Here's how the part is built. I have some questions about the finished solid (model axes, mm). A direction names the side the tool comes from. Round coordinates to 2 decimals unless told otherwise and drop trailing zeros. Write each loop counter-clockwise with the first axis right and the second up, starting at its lowest first coordinate (ties: lowest second). Pieces come first, ordered by that corner, then holes. Notation, with made-up numbers: (55, 34.5) - (80, 34.5) arc R24 ccw to (80, 72.5) - close; hole circle Ø4 at (3.5, 41.5). An arc over 180 degrees is marked (long way). Use one line per item in the form item = value. Start each with the question number.
1. I want a section at C-C, the plane x = -31. List the corners of the cut face in (y, z) for me.
2. We'd pull the mould along X, two halves only. Please class faces 5 (the flat face through (-12.7, -157, 6)), 6 (the flat face through (-159, -52.032, 6)), 7 (the cylindrical face through (-122.91, 115.86, 6.26)): +X half, -X half, draft (parallel to the pull), parting line (faces both ways), or undercut.
3. I want a section at A-A, the plane z = 5.25. List the corners of the cut face in (x, y) for me.
4. Which directions (+Z, -Z, +X, -X, +Y, -Y) give clear straight access to the entire face, cutting with the end or side of a thin tool? Please do faces 1 (the cylindrical face through (-9.48, 154.25, 7.04)), 2 (the flat face through (-163.83, -47, 6)), 3 (the flat face through (-160, -76.2, 6)), 4 (the flat face through (-6.35, -155, 9)).
5. I want a section at B-B, the plane x = -103.5. List the corners of the cut face in (y, z) for me, plus the area to 3 significant figures.
6. Will these pins go through, and if not, where does the flat tip stop? pin 1 (1 mm diameter, centred on y = -103, z = 6, fed in from -X); pin 2 (6.5 mm diameter, centred on x = -156, z = 4, fed in from -Y); pin 3 (1 mm diameter, centred on y = 95.5, z = 5, fed in from -X).
7. If I drill on line 1 along Y through (x, z) = (-8, 6.35); line 2 along Y through (x, z) = (-11, 6.35); line 3 along Y through (x, z) = (-14.5, 1), over which ranges is the centre line in solid material (lowest first)?
8. I want a section at D-D, the plane y = -3.5. List the corners of the cut face in (x, z) for me.
Autodesk Inventor part; units mm, degrees
ref_plane "YZ Plane" through (0, 0, 0) normal (1, 0, 0) x (0, 1, 0)
ref_plane "XZ Plane" through (0, 0, 0) normal (0, 1, 0) x (-1, 0, 0)
ref_plane "XY Plane" through (0, 0, 0) normal (0, 0, 1) x (1, 0, 0)
sketch "Sketch1" plane through (0, 0, 0) normal (0, 0, 1) x (1, 0, 0)
  arc A0 (-6.35, 145.9119) -> (0, -146.05) centre (0, 0) ccw
  line L0 (-168.91, 0) -> (168.91, 0) construction
  line L1 (0, -146.05) -> (0, -168.91) construction
  line L2 (-168.91, 0) -> (-168.91, -76.2)
  line L3 (-168.91, -76.2) -> (-150.7453, -76.2)
  line L4 (0, 0) -> (0, -47.2694) construction
  line L5 (0, -47.2694) -> (-158.75, -47.2694) construction
  line L6 (-158.75, -42.5069) -> (-153.67, -42.5069)
  line L7 (-153.67, -42.5069) -> (-153.67, -52.0319)
  line L8 (-153.67, -52.0319) -> (-163.83, -52.0319)
  line L9 (-163.83, -52.0319) -> (-163.83, -42.5069)
  line L10 (-163.83, -42.5069) -> (-158.75, -42.5069)
  arc A1 (-150.7453, -76.2) -> (-6.35, -168.7906) centre (0, 0) ccw
  arc A2 (-6.35, 168.7906) -> (-168.91, 0) centre (0, 0) ccw
  line L11 (-6.35, -145.9119) -> (-6.35, -151.13)
  line L12 (-6.35, -161.29) -> (-6.35, -168.7906)
  line L13 (-6.35, -145.9119) -> (-6.35, -151.13)
  line L14 (-6.35, -161.29) -> (-6.35, -168.7906)
  line L15 (-6.35, 168.7906) -> (-6.35, 161.29)
  line L16 (-6.35, 151.13) -> (-6.35, 145.9119)
  line L17 (-6.35, -168.7906) -> (-6.35, -161.29)
  line L18 (-6.35, -151.13) -> (-6.35, -145.9119)
  line L19 (-6.35, 161.29) -> (-6.35, 151.13)
  line L20 (-6.35, -151.13) -> (-6.35, -161.29)
  point P0 (0, 161.29)
  point P1 (0, -151.13)
  point P2 (0, -161.29)
  dimension "d0" = 292.1
  dimension "d8" = 76.2
  dimension "d9" = 47.2694
  dimension "d10" = 158.75
  dimension "d12" = 4.7625
  dimension "d13" = 5.08
  dimension "d14" = 9.525
  dimension "d15" = 10.16
  dimension "d17" = 5.08
  dimension "d22" = 22.8787
  dimension "d23" = 24.1681
  dimension "d26" = 168.91
extrude "Extrusion1" add sketch "Sketch1" along normal blind 12.7
sketch "Sketch2" plane through (-6.35, 145.9119, 0) normal (1, 0, 0) x (0, 0, -1)
  line L0 (0, 0) -> (0, 22.8787)
  line L1 (0, 22.8787) -> (-12.7, 22.8787)
  line L2 (0, 0) -> (-12.7, 0)
  circle A0 centre (-6.35, 11.436) radius 3.175
  line L3 (0, -145.9119) -> (96.3473, -145.9119) construction
  line L4 (96.3473, -145.9119) -> (-165.7611, -145.9119) construction
  circle A1 centre (-6.35, -303.2598) radius 3.175
  dimension "d27" = 6.35
  dimension "d28" = 11.4427
  dimension "d29" = 6.35
extrude "Extrusion2" cut sketch "Sketch2" against normal blind 6.35
properties part number "TopfemaleHoopSection_v3"
Model answer:
q1.outline = (-166.04, 0) - (-142.72, 0) - (-142.72, 12.7) - (-166.04, 12.7) - close; (142.72, 0) - (166.04, 0) - (166.04, 12.7) - (142.72, 12.7) - close
q2.face_5 = +X half
q2.face_6 = undercut
q2.face_7 = -X half
q3.outline = (-168.91, -76.2) - (-150.75, -76.2) arc R168.91 ccw to (-6.35, -168.79) - (-6.35, -160.33) - (-12.7, -160.33) - (-12.7, -154.37) - (-6.35, -154.37) - (-6.35, -145.91) arc R146.05 cw to (-6.35, 145.91) - (-6.35, 154.37) - (-12.7, 154.37) - (-12.7, 160.33) - (-6.35, 160.33) - (-6.35, 168.79) arc R168.91 ccw to (-168.91, 0) - close; hole (-163.83, -52.03) - (-153.67, -52.03) - (-153.67, -42.51) - (-163.83, -42.51) - close
q4.face_1 = +X
q4.face_2 = +Z, -Z
q4.face_3 = +Z, -Z, -X, -Y
q4.face_4 = +Z, -Z, +X, +Y, -Y
q5.outline = (-133.49, 0) - (-103.05, 0) - (-103.05, 12.7) - (-133.49, 12.7) - close; (103.05, 0) - (133.49, 0) - (133.49, 12.7) - (103.05, 12.7) - close
q5.area = 773 mm2
q6.pin_1 = -134.25
q6.pin_2 = -76.2
q6.pin_3 = -139.66
q7.line_1 = -168.72 to -160.52, -154.17 to -145.83, 145.83 to 154.17, 160.52 to 168.72
q7.line_2 = -168.55 to -160.52, -154.17 to -145.64, 145.64 to 154.17, 160.52 to 168.55
q7.line_3 = -168.29 to -145.33, 145.33 to 168.29
q8.outline = (-168.91, 0) - (-146.01, 0) - (-146.01, 12.7) - (-168.91, 12.7) - close
